Check sheet for the modelled part. Datum: model origin and axes. Units: mm. Give positions to 0.01 mm unless a question says otherwise; leave off trailing zeros. Answer as CSV lines item,"result". Start each with the question number.
(1) Material ranges on line 1 (X direction, y = 687.5, z = 8.5); line 2 (X direction, y = 549, z = 7.75), recorded low to high. Write a range as from..to.
(2) Gauge pin test, flat ends, axial feed: pin 1 Ø13 at (x, y) = (90, 597.5) entering from +Z; pin 2 Ø9 at (x, y) = (90, 372.5) entering from +Z (1 decimal). Record the tip position at first contact, or that the pin passes through.
(3) Section check A-A on z = 12.5. State how many separate pieces and enclosed holes the cut face has, plus the area to 3 significant figures.
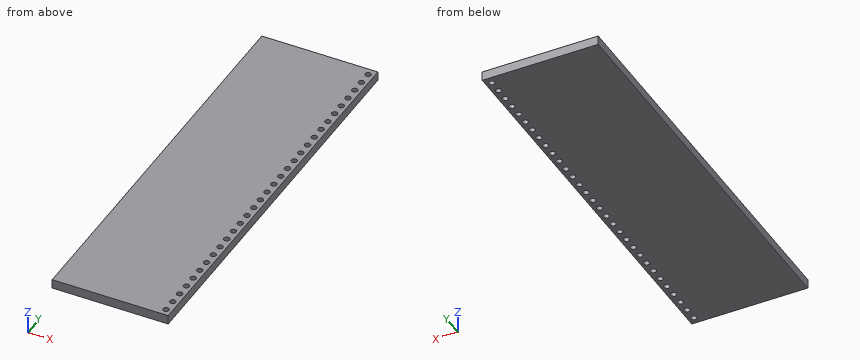
from build123d import *

# Parameters (mm, degrees)
SKETCH1_W           = 200
SKETCH1_H           = 700
BOSS_EXTRUDE1_DEPTH = 16
SKETCH2_OUTSIDE_W   = 347.638
SKETCH2_OUTSIDE_H   = 847.638
SKETCH2_OUTSIDE_R   = 5
CUT_EXTRUDE8_DEPTH  = 708.287777358
LPATTERN1_OUTLINE_R = 5
LPATTERN1_DEPTH     = 16


# Read off the part's stored shape, not the designer's step: LPattern1
with BuildPart() as part:
    # Sketch1 → Boss-Extrude1 (new body)
    with BuildSketch(Plane.XY):
        with Locations((0, 350)):
            Rectangle(SKETCH1_W, SKETCH1_H)
    extrude(amount=BOSS_EXTRUDE1_DEPTH)

    # Sketch2 outside → Cut-Extrude8 (cut, symmetric)
    # profile 1 of 2: a face of its own
    with BuildSketch(Plane.XY.offset(16)):
        with Locations((0, 350)):
            Rectangle(SKETCH2_OUTSIDE_W, SKETCH2_OUTSIDE_H)
        Polygon((90, 0), (100, 0), (100, 12.5), (100, 700), (-100, 700), (-100, 0), align=None, mode=Mode.SUBTRACT)
    # profile 2 of 2: a face of its own
    with BuildSketch(Plane.XY.offset(16)):
        with Locations(Location((90, 12.5, 0), (0, 0, 180))):
            Circle(SKETCH2_OUTSIDE_R)
    extrude(amount=CUT_EXTRUDE8_DEPTH, both=True, mode=Mode.SUBTRACT)

    # LPattern1 outline → LPattern1 (cut)
    with BuildSketch(Plane.XY):
        with Locations((90, 687.5)):
            Circle(LPATTERN1_OUTLINE_R)
        with Locations((90, 665)):
            Circle(LPATTERN1_OUTLINE_R)
        with Locations((90, 642.5)):
            Circle(LPATTERN1_OUTLINE_R)
        with Locations((90, 620)):
            Circle(LPATTERN1_OUTLINE_R)
        with Locations((90, 597.5)):
            Circle(LPATTERN1_OUTLINE_R)
        with Locations((90, 575)):
            Circle(LPATTERN1_OUTLINE_R)
        with Locations((90, 552.5)):
            Circle(LPATTERN1_OUTLINE_R)
        with Locations((90, 530)):
            Circle(LPATTERN1_OUTLINE_R)
        with Locations((90, 507.5)):
            Circle(LPATTERN1_OUTLINE_R)
        with Locations((90, 485)):
            Circle(LPATTERN1_OUTLINE_R)
        with Locations((90, 462.5)):
            Circle(LPATTERN1_OUTLINE_R)
        with Locations((90, 440)):
            Circle(LPATTERN1_OUTLINE_R)
        with Locations((90, 417.5)):
            Circle(LPATTERN1_OUTLINE_R)
        with Locations((90, 395)):
            Circle(LPATTERN1_OUTLINE_R)
        with Locations((90, 372.5)):
            Circle(LPATTERN1_OUTLINE_R)
        with Locations((90, 350)):
            Circle(LPATTERN1_OUTLINE_R)
        with Locations((90, 327.5)):
            Circle(LPATTERN1_OUTLINE_R)
        with Locations((90, 305)):
            Circle(LPATTERN1_OUTLINE_R)
        with Locations((90, 282.5)):
            Circle(LPATTERN1_OUTLINE_R)
        with Locations((90, 260)):
            Circle(LPATTERN1_OUTLINE_R)
        with Locations((90, 237.5)):
            Circle(LPATTERN1_OUTLINE_R)
        with Locations((90, 215)):
            Circle(LPATTERN1_OUTLINE_R)
        with Locations((90, 192.5)):
            Circle(LPATTERN1_OUTLINE_R)
        with Locations((90, 170)):
            Circle(LPATTERN1_OUTLINE_R)
        with Locations((90, 147.5)):
            Circle(LPATTERN1_OUTLINE_R)
        with Locations((90, 125)):
            Circle(LPATTERN1_OUTLINE_R)
        with Locations((90, 102.5)):
            Circle(LPATTERN1_OUTLINE_R)
        with Locations((90, 80)):
            Circle(LPATTERN1_OUTLINE_R)
        with Locations((90, 57.5)):
            Circle(LPATTERN1_OUTLINE_R)
        with Locations((90, 35)):
            Circle(LPATTERN1_OUTLINE_R)
    extrude(amount=LPATTERN1_DEPTH, mode=Mode.SUBTRACT)


solid = part.part
Working result:
1,line 1,"x = -100..85, 95..100"
1,line 2,"x = -100..86.43, 93.57..100"
2,pin 1,"stops at z = 16"
2,pin 2,"passes through"
3,separate pieces,"1"
3,enclosed holes,"31"
3,area,"138,000 mm^2"
